Could you check a few things on this drawing? It's one solid part, dimensions in mm from its lowest x, y, z. Give positions to 0.01 mm unless a question says otherwise; leave off trailing zeros. Order: outer loops, then holes, each group sorted by start corner. A loop starts at its lowest first (then second) coordinate and runs counter-clockwise, first axis right, second up.
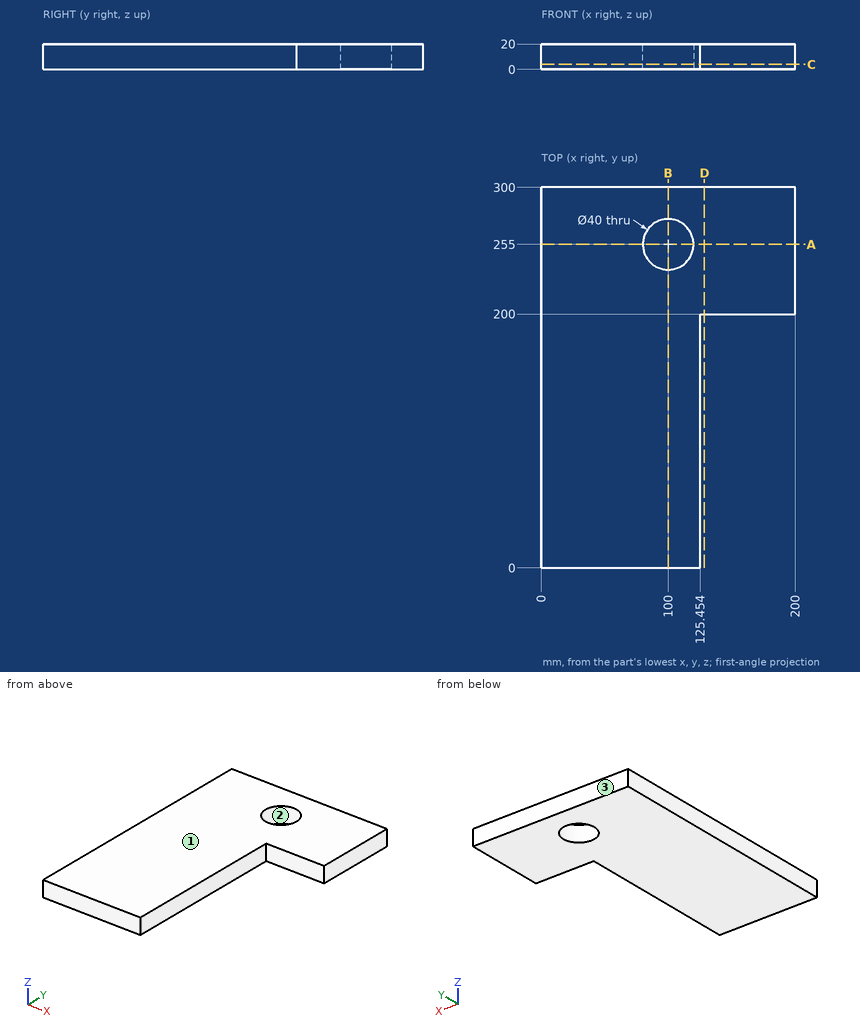
Q1. If we section it at C-C on z = 4: List the corners of the cut face in (x, y) for me.
Filled sheet:
outline: (0, 0) - (125.45, 0) - (125.45, 200) - (200, 200) - (200, 300) - (0, 300) - close; hole circle Ø40 at (100, 255)
Q2. Thinking about a two-plate mould opening in Y: for the marked faces 1, 2 and 3, which applies, released by +Y, released by -Y, zero draft, split by the parting line, or undercut?
Filled sheet:
face 1: zero draft
face 2: undercut
face 3: released by +Y
Q3. If we section it at D-D on x = 128.5: List the corners of the cut face in (y, z) for me.
Filled sheet:
outline: (200, 0) - (300, 0) - (300, 20) - (200, 20) - close
Q4. If we section it at B-B on x = 100: List the corners of the cut face in (y, z) for me.
Filled sheet:
outline: (0, 0) - (235, 0) - (235, 20) - (0, 20) - close; (275, 0) - (300, 0) - (300, 20) - (275, 20) - close
Q5. I'm going to push flat-ended pins straight in: P1, Ø10, axis at x = 159.5, z = 15, coming from the -Y side; P2, Ø10, axis at y = 75, z = 13.5, coming from the +X side. Where does each tip first touch, or does it pass through?
Filled sheet:
P1: stops at y = 200
P2: stops at x = 125.45
Q6. I need wall thicknesses on L1, parallel to Y at x = 100, z = 9.75; L2, parallel to X at y = 131, z = 8.25; L3, parallel to Y at x = 138.5, z = 16. Which ranges of each line are inside material? Lowest first, please.
Filled sheet:
L1: y = 0 to 235, 275 to 300
L2: x = 0 to 125.45
L3: y = 200 to 300
Q7. If we section it at A-A on y = 255: List the corners of the cut face in (x, z) for me.
Filled sheet:
outline: (0, 0) - (80, 0) - (80, 20) - (0, 20) - close; (120, 0) - (200, 0) - (200, 20) - (120, 20) - close
